Input: part model. Units: mm. Frame: model coordinates. A direction names the side the tool comes from. Coordinates: 2 decimals unless noted, no trailing zeros. Order: outer loops, then holes, each group sorted by start corner. A loop starts at its lowest first (then second) coordinate and runs counter-clockwise, first axis right, second up. Notation, with made-up numbers: (37, 56.5) -> (71, 56.5) arc R25 cw to (71, 76.5) -> close; hole circle Ø8 at (44, 46). An arc over 180 degrees is marked (long way). One line per item, written item: value. Start each with the question number.
from build123d import *

# Parameters (mm, degrees)
SKETCH2_R          = 2
CUT_EXTRUDE1_DEPTH = 112.579568022


with BuildPart() as part:
    # Sketch1 → Revolve1 (revolve)
    with BuildSketch(Plane.XY, mode=Mode.PRIVATE) as revolve1_sk:
        Polygon((-30, 25), (-30, 35), (-50, 35), (-50, 40), (-30, 40), (-30, 50), (-50, 50), (-50, 55), (-20, 55), (-20, 35), (-15, 35), (-15, 32), (15, 32), (15, 35), (20, 35), (20, 55), (30, 55), (30, 25), (0, 25), align=None)
    revolve(revolve1_sk.sketch.rotate(Axis((-97.55225871, 0, 0), (1, 0, 0)), 90), axis=Axis((-97.55225871, 0, 0), (1, 0, 0)))

    # Sketch2 → Cut-Extrude1 (cut, through all)
    with BuildSketch(Plane(origin=(30, 0, 0), x_dir=(0, 0, -1), z_dir=(1, 0, 0))):
        with Locations((26.450336353, 36.405764747)):
            Circle(SKETCH2_R)
        with Locations((42.797543233, 13.905764747)):
            Circle(SKETCH2_R)
        with Locations((0, 45)):
            Circle(SKETCH2_R)
        with Locations((42.797543233, -13.905764747)):
            Circle(SKETCH2_R)
        with Locations((26.450336353, -36.405764747)):
            Circle(SKETCH2_R)
        with Locations((0, -45)):
            Circle(SKETCH2_R)
        with Locations((-26.450336353, -36.405764747)):
            Circle(SKETCH2_R)
        with Locations((-42.797543233, -13.905764747)):
            Circle(SKETCH2_R)
        with Locations((-42.797543233, 13.905764747)):
            Circle(SKETCH2_R)
        with Locations((-26.450336353, 36.405764747)):
            Circle(SKETCH2_R)
    extrude(amount=-CUT_EXTRUDE1_DEPTH, mode=Mode.SUBTRACT)


solid = part.part
1) Access query for faces 4 (the flat face through (-20, -1, 36)), 5 (the cylindrical face through (25.07, 13.994, 44.796)), 6 (the flat face through (-30, -22, 34)). Directions: +Z, -Z, +X, -X, +Y, -Y. A direction counts if a zero-diameter tool reaches every point of the face in a straight line with its end or side. Return the directions, or none.
2) Section query D-D, the plane x = -17. Return the cut outline in (y, z), plus the area to 3 significant figures.
3) Mould query, pull axis X, two halves, no side actions, for faces 1 (the flat face through (-50, 35.4, 0.2)), 2 (the cylindrical face through (25.07, -38.18, -27.37)), 3 (the flat face through (15, 28.4, -15.4)). Classes: +X half, -X half, draft (parallel to the pull), parting line (faces both ways), or undercut.
4) Ray query, line 1 along Y through (x, z) = (27.5, 0); line 2 along Y through (x, z) = (-43.5, -11.5); line 3 along X through (y, z) = (-1, -46.5). Return the intervals inside material, ascending. Write a range as from..to.
5) Section query C-C, the plane z = 46.5. Return the cut outline in (x, y), plus the area to 3 significant figures.
6) Section query B-B, the plane y = -45. Return the cut outline in (x, z), plus the area to 3 significant figures.
7) Section query A-A, the plane x = -44.5. Return the cut outline in (y, z).
8) Pin query (flat end, axial travel): pin 1 Ø6 at (x, z) = (-37, -44) entering from -Y; pin 2 Ø5 at (y, z) = (-36.41, -26.45) entering from -X; pin 3 Ø8 at (x, z) = (5.5, 15.5) entering from -Y. Return the tip coordinate at first contact, or that it passes through.
Entries:
1. face 4: none
1. face 5: +X, -X
1. face 6: -X
2. outline: circle Ø70 at (0, 0); hole circle Ø50 at (0, 0)
2. area: 1,880 mm2
3. face 1: -X half
3. face 2: draft
3. face 3: undercut
4. line 1: y = -55..-47, -43..-25, 25..43, 47..55
4. line 2: y = -53.78..-48.66, -38.31..-33.06, 33.06..38.31, 48.66..53.78
4. line 3: x = -30..-20, 20..30
5. outline: (-50, -29.37) -> (-20, -29.37) -> (-20, 29.37) -> (-50, 29.37) -> (-50, 18.38) -> (-30, 18.38) -> (-30, -18.38) -> (-50, -18.38) -> close; (20, -29.37) -> (30, -29.37) -> (30, 29.37) -> (20, 29.37) -> close
5. area: 1,610 mm2
6. outline: (-50, -31.62) -> (-20, -31.62) -> (-20, -2) -> (-30, -2) -> (-30, -21.79) -> (-50, -21.79) -> close; (-50, 21.79) -> (-30, 21.79) -> (-30, 2) -> (-20, 2) -> (-20, 31.62) -> (-50, 31.62) -> close; (20, -31.62) -> (30, -31.62) -> (30, -2) -> (20, -2) -> close; (20, 2) -> (30, 2) -> (30, 31.62) -> (20, 31.62) -> close
6. area: 1,580 mm2
7. outline: circle Ø110 at (0, 0); circle Ø80 at (0, 0); hole circle Ø100 at (0, 0); hole circle Ø70 at (0, 0)
8. pin 1: stops at y = -36.66
8. pin 2: stops at x = -30
8. pin 3: stops at y = -29.86
